Input: part model. Units: mm. Frame: model coordinates. Face numbers are marked on the shaded views. A direction names the side the tool comes from. Give positions to 0.01 mm unless a question says otherwise; leave off trailing zeros. Order: outer loops, then holes, each group sorted by start corner. A loop starts at its lowest first (then second) coordinate and runs counter-clockwise, first axis right, second up. Notation, with made-up numbers: (26, -7) - (35, -7) arc R6 cw to (35, 3) - close; hole circle Ø2 at (39.5, 35.25). An arc over 180 degrees is marked (long way). Use a Markdown table: item, result.
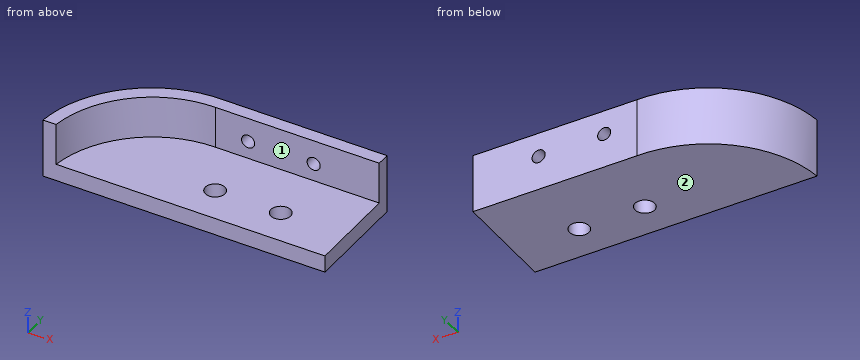
from build123d import *

# Parameters (mm, degrees)
SALIENTE_EXTRUIR1_DEPTH           = 4.5
CORTAR_EXTRUIR1_DEPTH             = 3.2
DI_METRO_DE_TALADRO_1_0_1_1_D     = 1
DI_METRO_DE_TALADRO_1_0_1_1_DEPTH = 8
DI_METRO_DE_TALADRO_1_5_1_5_1_D   = 1.5


with BuildPart() as part:
    # Croquis1 → Saliente-Extruir1 (new body)
    with BuildSketch(Plane.XY.offset(4.5)):
        with BuildLine():
            Line((-9, 0), (12.5, 0))
            Line((12.5, 0), (12.5, 8))
            Line((12.5, 8), (0, 8))
            ThreePointArc((0, 8), (-6.088245682, 5.786776392), (-9, 0))
        make_face()
    extrude(amount=-SALIENTE_EXTRUIR1_DEPTH)

    # Croquis2 → Cortar-Extruir1 (cut)
    with BuildSketch(Plane.XY.offset(4.5)):
        with BuildLine():
            Line((12.5, 7), (0, 7))
            ThreePointArc((0, 7), (-5.341079038, 5.032661758), (-8, 0))
            Line((-8, 0), (12.5, 0))
            Line((12.5, 0), (12.5, 7))
        make_face()
    extrude(amount=-CORTAR_EXTRUIR1_DEPTH, mode=Mode.SUBTRACT)

    # Diámetro de taladro Ø1.0 (1)1
    with Locations(Plane(origin=(0, 8, 0), x_dir=(1, 0, 0), z_dir=(0, 1, 0))):
        with Locations((2.5, -2.65), (7.5, -2.65)):
            Hole(DI_METRO_DE_TALADRO_1_0_1_1_D / 2, depth=DI_METRO_DE_TALADRO_1_0_1_1_DEPTH)

    # Diámetro de taladro Ø1.5 (1.5)1 (through all)
    with Locations(Plane.XY.offset(1.3)):
        with Locations((7.5, 2.75), (2.5, 2.75)):
            Hole(DI_METRO_DE_TALADRO_1_5_1_5_1_D / 2)


solid = part.part
1. Pin query (flat end, axial travel): pin 1 (1.4 mm diameter, centred on x = 2.5, y = 2.75, fed in from -Z); pin 2 (1 mm diameter, centred on x = 7.5, y = 5, fed in from +Z); pin 3 (2.5 mm diameter, centred on x = 6.5, z = 3, fed in from -Y); pin 4 (1 mm diameter, centred on x = 1.5, z = 2, fed in from +Y). Return the tip coordinate at first contact, or that it passes through.
Response:
| item | result |
|---|---|
| pin 1 | passes through |
| pin 2 | stops at z = 1.3 |
| pin 3 | stops at y = 7 |
| pin 4 | stops at y = 8 |
2. Material intervals for line 1 along Z through (x, y) = (2.5, 7.3); line 2 along Y through (x, z) = (7.5, 0.85); line 3 along Z through (x, y) = (7.25, 6), sorted ascending.
Response:
| item | result |
|---|---|
| line 1 | z = 0 to 2.15, 3.15 to 4.5 |
| line 2 | y = 0 to 2, 3.5 to 8 |
| line 3 | z = 0 to 1.3 |
3. Section query C-C (z = 0.75). Return loops of the section in (x, y), then the cut area to 3 significant figures.
Response:
| item | result |
|---|---|
| outline | (-9, 0) - (12.5, 0) - (12.5, 8) - (0, 8) arc R8.78 ccw to start; hole circle Ø1.5 at (2.5, 2.75); hole circle Ø1.5 at (7.5, 2.75) |
| area | 152 mm^2 |
4. Set-up query: the marked faces 1 and 2. Return all of +Z, -Z, +X, -X, +Y, -Y with unobstructed straight access to the full face (end or side cutting, diameter ignored); none if empty.
Response:
| item | result |
|---|---|
| face 1 | +Z, +X, -Y |
| face 2 | -Z, +X, -X, +Y, -Y |
5. Section query B-B (y = 3.25). Return loops of the section in (x, z), then the cut area to 3 significant figures.
Response:
| item | result |
|---|---|
| outline | (-8.06, 0) - (1.94, 0) - (1.94, 1.3) - (-6.86, 1.3) - (-6.86, 4.5) - (-8.06, 4.5) - close; (3.06, 0) - (6.94, 0) - (6.94, 1.3) - (3.06, 1.3) - close; (8.06, 0) - (12.5, 0) - (12.5, 1.3) - (8.06, 1.3) - close |
| area | 27.7 mm^2 |
6. Section query D-D (x = 6). Return loops of the section in (y, z), then the cut area to 3 significant figures.
Response:
| item | result |
|---|---|
| outline | (0, 0) - (8, 0) - (8, 4.5) - (7, 4.5) - (7, 1.3) - (0, 1.3) - close |
| area | 13.6 mm^2 |
7. Section query A-A (x = 2.5). Return loops of the section in (y, z).
Response:
| item | result |
|---|---|
| outline | (0, 0) - (2, 0) - (2, 1.3) - (0, 1.3) - close; (3.5, 0) - (8, 0) - (8, 2.15) - (7, 2.15) - (7, 1.3) - (3.5, 1.3) - close; (7, 3.15) - (8, 3.15) - (8, 4.5) - (7, 4.5) - close |
